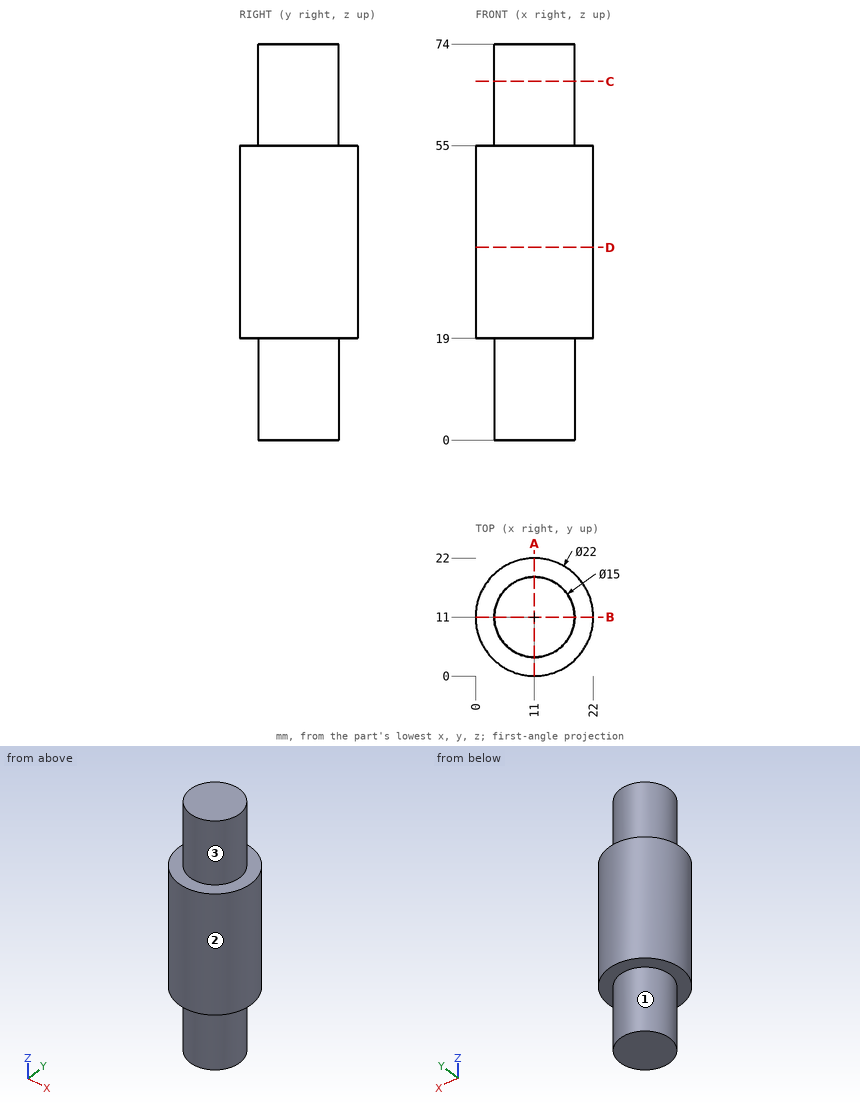
Geometry: see drawing. Coordinates: mm, zero at the bounding-box minimum. A direction names the side the tool comes from. Coordinates: 2 decimals unless noted, no trailing zeros. Loops run counter-clockwise (first coordinate to the right, second up) from the corner with the lowest first, then second, coordinate; pieces in that order, holes last.
Q1. Cut plane C-C (z = 67). Output: boundary loops of the cut face in (x, y).
Q2. Contact query for flat-ended pins moving along their axis: pin 1 (5 mm diameter, centred on x = 2.5, z = 59, fed in from +Y); pin 2 (12 mm diameter, centred on x = 18, z = 20.5, fed in from +Y); pin 3 (6 mm diameter, centred on x = 3.5, z = 12, fed in from +Y). Output: stop coordinate, or through.
Q3. Material intervals for line 1 (Z direction, x = 2, y = 8.75); line 2 (X direction, y = 4, z = 22); line 3 (X direction, y = 11.75, z = 25), sorted ascending.
Q4. Cut plane D-D (z = 36). Output: boundary loops of the cut face in (x, y), then the cut area to 3 significant figures.
Q5. Cut plane A-A (x = 11). Output: boundary loops of the cut face in (y, z), then the cut area to 3 significant figures.
Q6. Set-up query: the marked faces 1, 2 and 3. Return all of +Z, -Z, +X, -X, +Y, -Y with unobstructed straight access to the full face (end or side cutting, diameter ignored); none if empty.
Working result:
1. outline: circle Ø15 at (11, 11)
2. pin 1: stops at y = 15.5
2. pin 2: stops at y = 21.95
2. pin 3: stops at y = 17
3. line 1: z = 19 to 55
3. line 2: x = 2.51 to 19.49
3. line 3: x = 0.03 to 21.97
4. outline: circle Ø22 at (11, 11)
4. area: 380 mm2
5. outline: (0, 19) - (3.5, 19) - (3.5, 0) - (18.5, 0) - (18.5, 19) - (22, 19) - (22, 55) - (18.5, 55) - (18.5, 74) - (3.5, 74) - (3.5, 55) - (0, 55) - close
5. area: 1,360 mm2
6. face 1: -Z
6. face 2: +Z, -Z
6. face 3: +Z
